Source: CAD feature listing. Evaluate the final solid. Frame: model axes, mm. A direction names the side the tool comes from. Round coordinates to 2 decimals unless told otherwise and drop trailing zeros. Write each loop counter-clockwise with the first axis right and the second up, starting at its lowest first coordinate (ties: lowest second). Pieces come first, ordered by that corner, then holes. Notation, with made-up numbers: M -35,-30.5 L -5,-30.5 A11 cw -5,-26.5 Z; hole C 40.5,74.25 d5. An arc over 180 degrees is marked long. Answer in a Markdown table with one row per item.
from build123d import *

# Parameters (mm, degrees)
SKETCH1_W           = 20
SKETCH1_H           = 5
BOSS_EXTRUDE1_DEPTH = 1
SKETCH1_3_W         = 20
SKETCH1_3_H         = 5
SKETCH1_3_W_2       = 18
SKETCH1_3_H_2       = 3
SKETCH1_3_R         = 1
BOSS_EXTRUDE2_DEPTH = 1


with BuildPart() as part:
    # Sketch1 → Boss-Extrude1 (new body)
    with BuildSketch(Plane(origin=(0, 0, 0), x_dir=(1, 0, 0), z_dir=(0, 1, 0))):
        Rectangle(SKETCH1_W, SKETCH1_H)
    extrude(amount=BOSS_EXTRUDE1_DEPTH)

    # Sketch1_3 → Boss-Extrude2 (add)
    with BuildSketch(Plane(origin=(0, 0, 0), x_dir=(1, 0, 0), z_dir=(0, 1, 0))):
        Rectangle(SKETCH1_3_W, SKETCH1_3_H)
        Rectangle(SKETCH1_3_W_2, SKETCH1_3_H_2, mode=Mode.SUBTRACT)
        with Locations((-5, 0)):
            Circle(SKETCH1_3_R)
        Circle(SKETCH1_3_R)
        with Locations((5, 0)):
            Circle(SKETCH1_3_R)
    extrude(amount=-BOSS_EXTRUDE2_DEPTH)


solid = part.part
Q1. Material intervals for probe 1 along Z at (x, y) = (0, -0.1); probe 2 along Z at (x, y) = (1.75, -0.35); probe 3 along X at (y, z) = (-0.4, -0.15), sorted ascending.
Solutions:
| item | result |
|---|---|
| probe 1 | z = -2.5 to -1.5, -1 to 1, 1.5 to 2.5 |
| probe 2 | z = -2.5 to -1.5, 1.5 to 2.5 |
| probe 3 | x = -10 to -9, -5.99 to -4.01, -0.99 to 0.99, 4.01 to 5.99, 9 to 10 |
Q2. Section D-D (x = 5.25). Return loops of the section in (y, z), and give its area (3 significant figures).
Solutions:
| item | result |
|---|---|
| outline | M -1,-2.5 L 1,-2.5 L 1,2.5 L -1,2.5 L -1,1.5 L 0,1.5 L 0,0.97 L -1,0.97 L -1,-0.97 L 0,-0.97 L 0,-1.5 L -1,-1.5 Z |
| area | 8.94 mm2 |
Q3. Access query for faces 4 (the flat face through (5, -1, 0)), 5 (the flat face through (9, -0.5, 0)). Directions: +Z, -Z, +X, -X, +Y, -Y. A direction counts if a zero-diameter tool reaches every point of the face in a straight line with its end or side. Return the directions, or none.
Solutions:
| item | result |
|---|---|
| face 4 | +Z, -Z, +X, -X, -Y |
| face 5 | -Y |
Q4. Section B-B (z = 0). Return loops of the section in (x, y), and give its area (3 significant figures).
Solutions:
| item | result |
|---|---|
| outline | M -10,-1 L -9,-1 L -9,0 L -6,0 L -6,-1 L -4,-1 L -4,0 L -1,0 L -1,-1 L 1,-1 L 1,0 L 4,0 L 4,-1 L 6,-1 L 6,0 L 9,0 L 9,-1 L 10,-1 L 10,1 L -10,1 Z |
| area | 28.0 mm2 |
Q5. Pull-direction query (Z, two-part tool) for faces 1 (the flat face through (0, 0, 2.5)), 2 (the flat face through (-0.1, 0, 1.3)), 3 (the flat face through (10, 0, 0)); classes: pulls with the +Z half, pulls with the -Z half, needs draft (parallel to the pull), parting line crosses it, or undercut.
Solutions:
| item | result |
|---|---|
| face 1 | pulls with the +Z half |
| face 2 | undercut |
| face 3 | needs draft |
Q6. Section C-C (x = -5). Return loops of the section in (y, z).
Solutions:
| item | result |
|---|---|
| outline | M -1,-2.5 L 1,-2.5 L 1,2.5 L -1,2.5 L -1,1.5 L 0,1.5 L 0,1 L -1,1 L -1,-1 L 0,-1 L 0,-1.5 L -1,-1.5 Z |
